For this review, take the finished solid that the model builds, in its own axes (mm). Face numbers are marked on the shaded views. A direction names the side the tool comes from. Give positions to 0.01 mm unless a question says otherwise; leave off trailing zeros. Write each loop counter-clockwise with the first axis right and the second up, starting at its lowest first coordinate (ties: lowest second). Pieces come first, ordered by that corner, then holes.
1) We need section C-C on x = 25. Give the boundary of the cut face in (y, z).
2) Draft analysis for pull direction X (two halves, no side actions). For the marked faces 1, 2 and 3, state which applies: pulls with the +X half, pulls with the -X half, needs draft (parallel to the pull), parting line crosses it, or undercut.
3) Wall thickness on line 1 along X through (y, z) = (7.25, 2.5); line 2 along X through (y, z) = (7.5, 6.25); line 3 along X through (y, z) = (4, 3.5): over which ranges is each line inside the solid? List them lowest first.
4) Machinability: for the marked faces 4, 5 and 6, which of the approach directions +Z, -Z, +X, -X, +Y, -Y give a long, thin tool a straight path to every point of the face, cutting with its end or side? Answer none if there is none.
5) We need section B-B on y = 6.5. Give the number of separate pieces and of enclosed holes in the cut face, and give its area (3 significant figures).
6) We need section A-A on x = 38.25. Give the boundary of the cut face in (y, z), and give its area (4 significant figures).
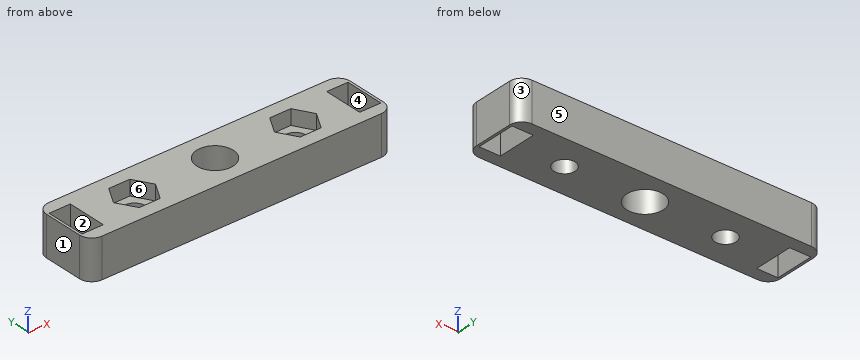
from build123d import *

# Parameters (mm, degrees)
SKETCH_1_W          = 50
SKETCH_1_H          = 10.5
EXTRUDE_1_DEPTH     = 17
SKETCH_2_W          = 36
SKETCH_2_H          = 3.5
CUT_EXTRUDE_1_DEPTH = 10
CUT_EXTRUDE_2_DEPTH = 10.5
SKETCH_4_W          = 3.5
SKETCH_4_H          = 6.5
CUT_EXTRUDE_3_DEPTH = 6.5
FILLET_1_R          = 2
SKETCH_6_R          = 3
SKETCH_6_R_2        = 1.75
CUT_EXTRUDE_4_DEPTH = 18
CUT_EXTRUDE_5_DEPTH = 11
CUT_EXTRUDE_6_DEPTH = 3
SKETCH_9_W          = 58.421136066
SKETCH_9_H          = 24.245128271
CUT_EXTRUDE_7_DEPTH = 11.5


with BuildPart() as part:
    # ｽｹｯﾁ1 → ﾎﾞｽ - 押し出し1 (new body)
    with BuildSketch(Plane.XY):
        with Locations((25, 5.25)):
            Rectangle(SKETCH_1_W, SKETCH_1_H)
    extrude(amount=EXTRUDE_1_DEPTH)

    # ｽｹｯﾁ2 → ｶｯﾄ - 押し出し1 (cut)
    with BuildSketch(Plane.XY.offset(17)):
        with Locations((25, 5.25)):
            Rectangle(SKETCH_2_W, SKETCH_2_H)
    extrude(amount=-CUT_EXTRUDE_1_DEPTH, mode=Mode.SUBTRACT)

    # ｽｹｯﾁ3 → ｶｯﾄ - 押し出し2 (cut)
    with BuildSketch(Plane.XZ):
        Polygon((1, 17), (3, 12), (7, 12), (17, 17), align=None)
        Polygon((33, 17), (43, 12), (47, 12), (49, 17), align=None)
    extrude(amount=-CUT_EXTRUDE_2_DEPTH, mode=Mode.SUBTRACT)

    # ｽｹｯﾁ4 → ｶｯﾄ - 押し出し3 (cut)
    with BuildSketch(Plane(origin=(0, 0, 0), x_dir=(-1, 0, 0), z_dir=(0, 0, -1))):
        with Locations((-2.15, 5.25)):
            Rectangle(SKETCH_4_W, SKETCH_4_H)
        with Locations((-47.85, 5.25)):
            Rectangle(SKETCH_4_W, SKETCH_4_H)
    extrude(amount=-CUT_EXTRUDE_3_DEPTH, mode=Mode.SUBTRACT)

    # ﾌｨﾚｯﾄ1
    fillet_1_edges = [part.edges().sort_by_distance(p)[0] for p in [
        (0, 0, 8.5),
        (0, 10.5, 8.5),
        (50, 0, 8.5),
        (50, 10.5, 8.5),
    ]]
    fillet(fillet_1_edges, radius=FILLET_1_R)

    # ｽｹｯﾁ6 → ｶｯﾄ - 押し出し4 (cut, through all)
    with BuildSketch(Plane(origin=(0, 0, 0), x_dir=(-1, 0, 0), z_dir=(0, 0, -1))):
        with Locations((-25, 5.25)):
            Circle(SKETCH_6_R)
        with Locations((-11.75, 5.25)):
            Circle(SKETCH_6_R_2)
        with Locations((-38.25, 5.25)):
            Circle(SKETCH_6_R_2)
    extrude(amount=-CUT_EXTRUDE_4_DEPTH, mode=Mode.SUBTRACT)

    # ｽｹｯﾁ7 → ｶｯﾄ - 押し出し5 (cut, through all)
    with BuildSketch(Plane.XY.offset(7)):
        Polygon((34.785898385, 5.25), (36.517949192, 2.25), (39.982050808, 2.25), (41.714101615, 5.25), (39.982050808, 8.25), (36.517949192, 8.25), align=None)
        Polygon((13.482050808, 8.25), (15.214101615, 5.25), (13.482050808, 2.25), (10.017949192, 2.25), (8.285898385, 5.25), (10.017949192, 8.25), align=None)
    extrude(amount=CUT_EXTRUDE_5_DEPTH, mode=Mode.SUBTRACT)

    # ｽｹｯﾁ8 → ｶｯﾄ - 押し出し6 (cut)
    with BuildSketch(Plane.XY.offset(7)):
        Polygon((36.517949192, 2.25), (39.982050808, 2.25), (41.714101615, 5.25), (39.982050808, 8.25), (36.517949192, 8.25), (34.785898385, 5.25), align=None)
        Polygon((15.214101615, 5.25), (13.482050808, 2.25), (10.017949192, 2.25), (8.285898385, 5.25), (10.017949192, 8.25), (13.482050808, 8.25), align=None)
    extrude(amount=-CUT_EXTRUDE_6_DEPTH, mode=Mode.SUBTRACT)

    # ｽｹｯﾁ9 → ｶｯﾄ - 押し出し7 (cut, through all)
    with BuildSketch(Plane(origin=(0, 0, 6.5), x_dir=(-1, 0, 0), z_dir=(0, 0, -1))):
        with Locations((-24.970881096, 5.810967265)):
            Rectangle(SKETCH_9_W, SKETCH_9_H)
    extrude(amount=-CUT_EXTRUDE_7_DEPTH, mode=Mode.SUBTRACT)


solid = part.part
Results list:
1. outline: (0, 0) - (2.25, 0) - (2.25, 6.5) - (0, 6.5) - close; (8.25, 0) - (10.5, 0) - (10.5, 6.5) - (8.25, 6.5) - close
2. face 1: pulls with the -X half
2. face 2: undercut
2. face 3: pulls with the +X half
3. line 1: x = 0 to 0.4, 3.9 to 22.76, 27.24 to 46.1, 49.6 to 50
3. line 2: x = 0 to 0.4, 3.9 to 9.58, 13.92 to 23.02, 26.98 to 36.08, 40.42 to 46.1, 49.6 to 50
3. line 3: x = 0 to 0.4, 3.9 to 10.53, 12.97 to 22.27, 27.73 to 37.03, 39.47 to 46.1, 49.6 to 50
4. face 4: +Z, -Z
4. face 5: +Z, -Z, +X, -X, +Y
4. face 6: +Z
5. separate pieces: 6
5. enclosed holes: 0
5. area: 197 mm2
6. outline: (0, 0) - (3.5, 0) - (3.5, 4) - (2.25, 4) - (2.25, 6.5) - (0, 6.5) - close; (7, 0) - (10.5, 0) - (10.5, 6.5) - (8.25, 6.5) - (8.25, 4) - (7, 4) - close
6. area: 39.25 mm2
